from build123d import *

# Parameters (mm, degrees)
F0_W     = 100
F0_H     = 90
F1_DEPTH = 3
F3_D     = 4.8
F3_DEPTH = 10
F4_R     = 5
F6_D     = 62
F6_DEPTH = 10


with BuildPart() as f1:
    # F0 (on Front) → F1 (new body)
    with BuildSketch(Plane.XZ):
        with Locations((-1726.19823, -1534.163168)):
            Rectangle(F0_W, F0_H)
    extrude(amount=F1_DEPTH)

    # F3
    with Locations(Plane.XZ.offset(3)):
        with Locations((-1771.19823, -1494.163168), (-1681.19823, -1494.163168), (-1681.19823, -1574.163168), (-1771.19823, -1574.163168)):
            Hole(F3_D / 2, depth=F3_DEPTH)

    # F4
    f4_edges = [f1.edges().sort_by_distance(p)[0] for p in [
        (-1676.19823, -1.5, -1489.163168),
        (-1676.19823, -1.5, -1579.163168),
        (-1776.19823, -1.5, -1489.163168),
        (-1776.19823, -1.5, -1579.163168),
    ]]
    fillet(f4_edges, radius=F4_R)

    # F6
    with Locations(Plane.XZ.offset(3)):
        with Locations((-1726.19823, -1534.163168)):
            Hole(F6_D / 2, depth=F6_DEPTH)


solid = f1.part
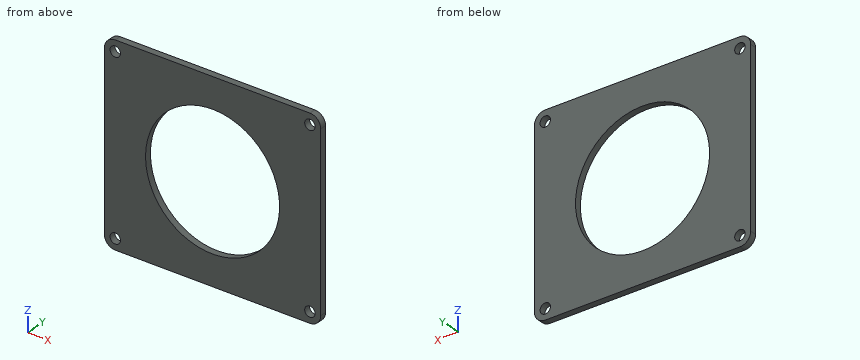
Design review of the part built by this model. Coordinates are the model's own, in mm. Give positions to 0.01 mm unless a question says otherwise; leave off trailing zeros. Loops run counter-clockwise (first coordinate to the right, second up) from the corner with the lowest first, then second, coordinate; pieces in that order, holes last. Notation, with made-up numbers: (73.25, 75) - (123.25, 75) arc R15 cw to (123.25, 88) - close; hole circle Ø6 at (61, -38). An arc over 180 degrees is marked (long way). Write item = value, one per line.
1) Take a section at B-B on x = -1698. State the section outline as (y, z) points, and give its area (3 significant figures).
Result sheet:
outline = (-3, -1579.16) - (0, -1579.16) - (0, -1547.04) - (-3, -1547.04) - close; (-3, -1521.28) - (0, -1521.28) - (0, -1489.16) - (-3, -1489.16) - close
area = 193 mm2
2) Take a section at C-C on y = -0.95. State the section outline as (x, z) points, and give its area (3 significant figures).
Result sheet:
outline = (-1776.2, -1574.16) arc R5 ccw to (-1771.2, -1579.16) - (-1681.2, -1579.16) arc R5 ccw to (-1676.2, -1574.16) - (-1676.2, -1494.16) arc R5 ccw to (-1681.2, -1489.16) - (-1771.2, -1489.16) arc R5 ccw to (-1776.2, -1494.16) - close; hole circle Ø4.8 at (-1771.2, -1574.16); hole circle Ø4.8 at (-1771.2, -1494.16); hole circle Ø62 at (-1726.2, -1534.16); hole circle Ø4.8 at (-1681.2, -1574.16); hole circle Ø4.8 at (-1681.2, -1494.16)
area = 5,890 mm2
3) To check wall thickness, follow line 1 (X direction, y = -2.55, z = -1493); line 2 (Z direction, x = -1769, y = -0.55); line 3 (Z direction, x = -1739.5, y = -1.4). State the ranges of each line that lie inside material, in increasing order.
Result sheet:
line_1 = -1776.06 to -1773.3, -1769.1 to -1683.3, -1679.1 to -1676.34
line_2 = -1579.16 to -1575.13, -1573.2 to -1495.13, -1493.2 to -1489.16
line_3 = -1579.16 to -1562.16, -1506.16 to -1489.16
4) Clearance check with a flat-ended pin moving along its axis: pin 1 Ø3 at (x, z) = (-1681.2, -1494.16) entering from -Y. State where the tip first meets the part, or that it passes through.
Result sheet:
pin_1 = through
5) Take a section at A-A on z = -1536. State the section outline as (x, y) points.
Result sheet:
outline = (-1776.2, -3) - (-1757.14, -3) - (-1757.14, 0) - (-1776.2, 0) - close; (-1695.25, -3) - (-1676.2, -3) - (-1676.2, 0) - (-1695.25, 0) - close
